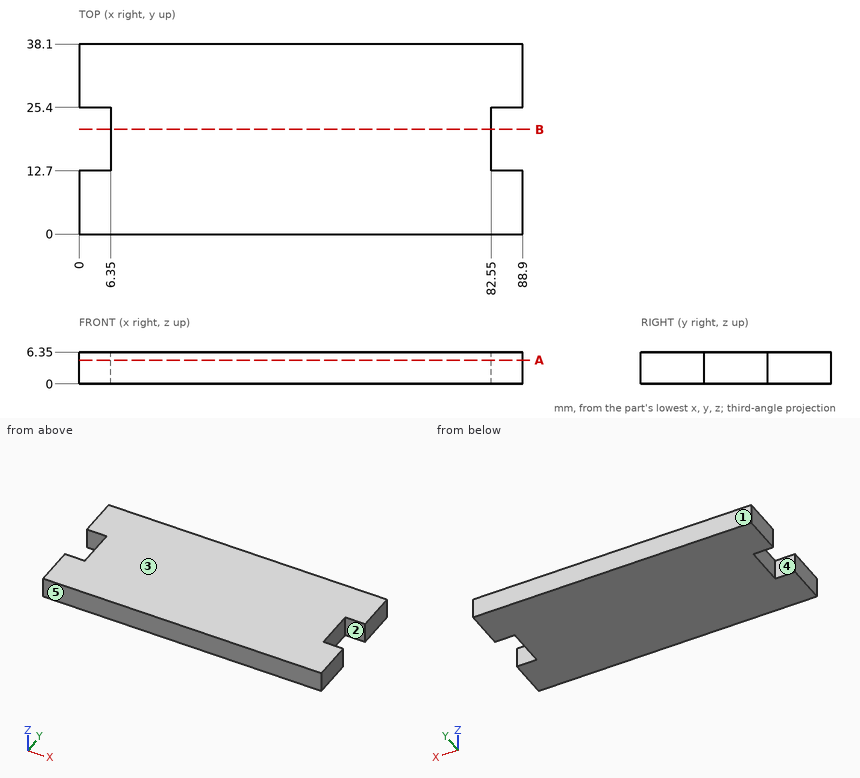
Design review of the part shown in the three views and the two pictorial views. Dimensions are in mm from the part's minimum x, y and z. A direction names the side the tool comes from. Round coordinates to 2 decimals unless told otherwise and drop trailing zeros. Loops run counter-clockwise (first coordinate to the right, second up) from the corner with the lowest first, then second, coordinate; pieces in that order, holes last. Notation, with made-up numbers: (12.5, -39.75) -> (18.5, -39.75) arc R17 ccw to (18.5, -12.75) -> close; hole circle Ø2 at (23, 74.5). An arc over 180 degrees is marked (long way). Use one line per item in the form item = value. Start each with the question number.
Q1. We need section A-A on z = 4.75. Give the boundary of the cut face in (x, y), then the cut area to 3 significant figures.
Q2. Draft analysis for pull direction Y (two halves, no side actions). For the marked faces 3, 4 and 5, state which applies: +Y half, -Y half, draft (parallel to the pull), parting line (faces both ways), or undercut.
Q3. Machinability: for the marked faces 1 and 2, which of the approach directions +Z, -Z, +X, -X, +Y, -Y give a long, thin tool a straight path to every point of the face, cutting with its end or side? Answer none if there is none.
Q4. For pin 1 Ø1.9 at (y, z) = (20, 3) entering from +X; pin 2 Ø3 at (y, z) = (18, 2) entering from -X, all flat-tipped, find the tip position at first contact; note any pin that passes through.
Q5. We need section B-B on y = 21. Give the boundary of the cut face in (x, z).
Q6. Wall thickness on line 1 along X through (y, z) = (21, 4): over which ranges is the line inside the solid? List them lowest first. Write a range as [from, to].
Calculated:
q1.outline = (0, 0) -> (88.9, 0) -> (88.9, 12.7) -> (82.55, 12.7) -> (82.55, 25.4) -> (88.9, 25.4) -> (88.9, 38.1) -> (0, 38.1) -> (0, 25.4) -> (6.35, 25.4) -> (6.35, 12.7) -> (0, 12.7) -> close
q1.area = 3,230 mm²
q2.face_3 = draft
q2.face_4 = undercut
q2.face_5 = -Y half
q3.face_1 = +Z, -Z, +X, -X, +Y
q3.face_2 = +Z, -Z, +X
q4.pin_1 = 82.55
q4.pin_2 = 6.35
q5.outline = (6.35, 0) -> (82.55, 0) -> (82.55, 6.35) -> (6.35, 6.35) -> close
q6.line_1 = [6.35, 82.55]
